For this review, take the finished solid that the model builds, in its own axes (mm). Face numbers are marked on the shaded views. A direction names the side the tool comes from. Give positions to 0.01 mm unless a question says otherwise; leave off trailing zeros. Order: outer loops, then holes, each group sorted by start corner. A loop starts at its lowest first (then second) coordinate and runs counter-clockwise, first axis right, second up. Notation, with made-up numbers: M 7,37 L 18,37 A19 ccw 18,56 Z; hole C 25.5,50.5 d4. An arc over 180 degrees is marked long. Use CSV: the item, a comma, the result in double quotes. Start each with the question number.
(1) Clearance check with flat-ended pins moving along their axes: P1, Ø4, axis at x = -18.5, z = -5.5, coming from the -Y side; P2, Ø4, axis at x = -21, y = 182, coming from the +Z side; P3, Ø12, axis at y = 46.5, z = 10, coming from the -X side; P4, Ø5, axis at x = 11.5, y = 142, coming from the +Z side. State where each tip first meets the part, or that it passes through.
(2) Consider section A-A (y = 134.5). Write out the cut boundary in (x, z), and give its area (3 significant figures).
(3) Draft analysis for pull direction Y (two halves, no side actions). For the marked faces 4, 5 and 6, state which applies: pulls with the +Y half, pulls with the -Y half, needs draft (parallel to the pull), parting line crosses it, or undercut.
(4) Wall thickness on L1, parallel to Y at x = 23.5, z = 26.5; L2, parallel to Z at x = 1.5, y = 120.5; L3, parallel to Z at x = -14, y = 102: over which ranges is each line inside the solid? List them lowest first. Write a range as from..to.
(5) Tool access review of the marked faces 1, 2 and 3: name each direction out of +Z, -Z, +X, -X, +Y, -Y from which nothing blocks a thin tool from reaching the whole face with its end or side.
```python
from build123d import *

# Parameters (mm, degrees)
SKETCH2_R           = 35
BOSS_EXTRUDE1_DEPTH = 200
SKETCH3_R           = 15
BOSS_EXTRUDE2_DEPTH = 95
FILLET1_R           = 20
FILLET2_R           = 10
BOSS_EXTRUDE3_START = 1
SKETCH4_R           = 16
BOSS_EXTRUDE3_DEPTH = 60
BOSS_EXTRUDE4_START = -30
SKETCH5_R           = 35.5
BOSS_EXTRUDE4_DEPTH = 50


with BuildPart() as part:
    # Sketch2 → Boss-Extrude1 (new body)
    with BuildSketch(Plane(origin=(0, 0, 0), x_dir=(1, 0, 0), z_dir=(0, 1, 0))):
        with Locations(Location((0, 0, 0), (0, 0, 270))):
            Circle(SKETCH2_R)
    extrude(amount=BOSS_EXTRUDE1_DEPTH)

    # Sketch3 → Boss-Extrude2 (add)
    with BuildSketch(Plane(origin=(0, 200, 0), x_dir=(1, 0, 0), z_dir=(0, 1, 0))):
        with Locations(Location((0, 0, 0), (0, 0, 270))):
            Circle(SKETCH3_R)
    extrude(amount=BOSS_EXTRUDE2_DEPTH)

    # Fillet1
    fillet1_edges = [part.edges().sort_by_distance(p)[0] for p in [
        (0, 200, -15),
    ]]
    fillet(fillet1_edges, radius=FILLET1_R - 0.0001)  # a hair under: the kernel refuses the full size

    # Fillet2
    fillet2_edges = [part.edges().sort_by_distance(p)[0] for p in [
        (0, 200, -35),
    ]]
    fillet(fillet2_edges, radius=FILLET2_R)

    # Sketch4 → Boss-Extrude3 (add)
    with BuildSketch(Plane(origin=(0, 295, 0), x_dir=(1, 0, 0), z_dir=(0, 1, 0)).offset(BOSS_EXTRUDE3_START)):
        with Locations(Location((0, 0, 0), (0, 0, 270))):
            Circle(SKETCH4_R)
    extrude(amount=-BOSS_EXTRUDE3_DEPTH)

    # Sketch5 → Boss-Extrude4 (add)
    with BuildSketch(Plane.XZ.offset(BOSS_EXTRUDE4_START)):
        with Locations(Location((0, 0, 0), (0, 0, 270))):
            Circle(SKETCH5_R)
    extrude(amount=-BOSS_EXTRUDE4_DEPTH)


solid = part.part
```
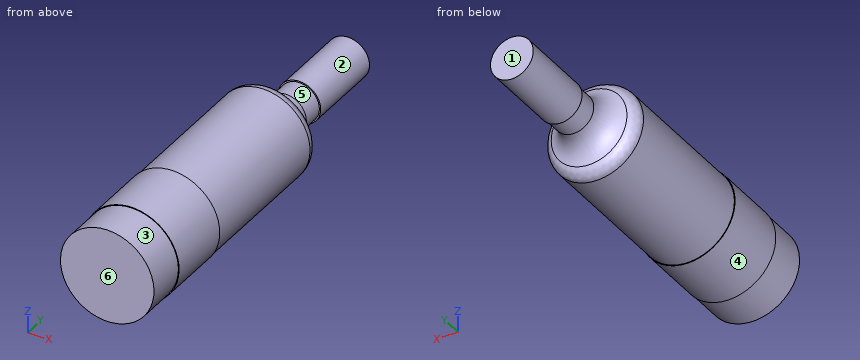
Check result:
1,P1,"stops at y = 0"
1,P2,"stops at z = 29.39"
1,P3,"stops at x = -35.27"
1,P4,"stops at z = 33.82"
2,outline,"C 0,0 d70"
2,area,"3,850 mm^2"
3,face 4,"needs draft"
3,face 5,"undercut"
3,face 6,"pulls with the -Y half"
4,L1,"y = 30..80"
4,L2,"z = -34.97..34.97"
4,L3,"z = -32.08..32.08"
5,face 1,"+Z, -Z, +X, -X, +Y"
5,face 2,"+Y"
5,face 3,"-Y"
